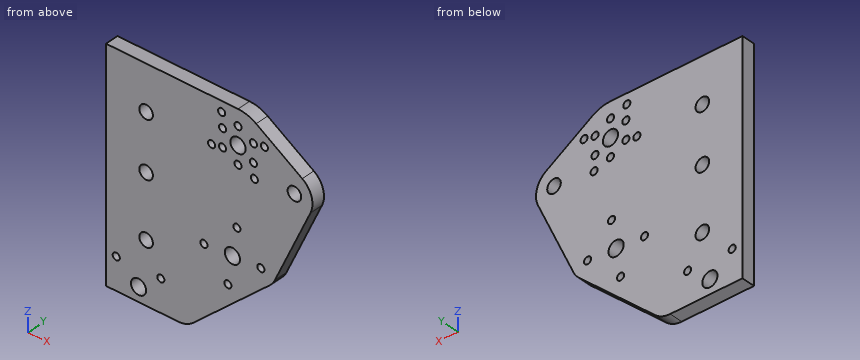
from build123d import *

# Parameters (mm, degrees)
ESBO_O1_R                = 3.4
ESBO_O1_R_2              = 1.6
ESBO_O1_R_3              = 3.05
RESSALTO_EXTRUS_O1_DEPTH = 6
ESBO_O2_R                = 3.05
CORTE_EXTRUS_O1_DEPTH    = 10


with BuildPart() as part:
    # Esboço1 → Ressalto-extrusão1 (new body)
    with BuildSketch(Plane.XZ.offset(6)):
        with BuildLine():
            ThreePointArc((148.858963728, -17.550205761), (150.213387743, -16.041631797), (151.235707119, -14.290882553))
            Line((151.235707119, -14.290882553), (167.194797105, 20.786465148))
            ThreePointArc((167.194797105, 20.786465148), (167.685761217, 27.75097204), (163.500492356, 33.339256802))
            Line((163.500492356, 33.339256802), (142.828800476, 46.629357452))
            ThreePointArc((142.828800476, 46.629357452), (138.919886426, 48.415130742), (134.666145804, 49.026919929))
            Line((134.666145804, 49.026919929), (75.43742995, 49.026919929))
            Line((75.43742995, 49.026919929), (75.43742995, -51.3))
            Line((75.43742995, -51.3), (107.856417314, -51.3))
            ThreePointArc((107.856417314, -51.3), (111.461591333, -50.627524875), (114.581887382, -48.700544058))
            Line((114.581887382, -48.700544058), (148.858963728, -17.550205761))
        make_face()
        with Locations(Location((90.03742995, -45, 0), (0, 0, 270))):
            Circle(ESBO_O1_R, mode=Mode.SUBTRACT)
        with Locations(Location((80.03742995, -37, 0), (0, 0, 270))):
            Circle(ESBO_O1_R_2, mode=Mode.SUBTRACT)
        with Locations(Location((100.03742995, -37, 0), (0, 0, 270))):
            Circle(ESBO_O1_R_2, mode=Mode.SUBTRACT)
        with Locations(Location((119.376459837, -13.805034822, 0), (0, 0, 270))):
            Circle(ESBO_O1_R_2, mode=Mode.SUBTRACT)
        with Locations(Location((130.137211947, -25.645905315, 0), (0, 0, 270))):
            Circle(ESBO_O1_R_2, mode=Mode.SUBTRACT)
        with Locations(Location((132.15737995, -13, 0), (0, 0, 270))):
            Circle(ESBO_O1_R, mode=Mode.SUBTRACT)
        with Locations(Location((144.938300063, -12.194965178, 0), (0, 0, 270))):
            Circle(ESBO_O1_R_2, mode=Mode.SUBTRACT)
        with Locations(Location((134.177547953, -0.354094685, 0), (0, 0, 270))):
            Circle(ESBO_O1_R_2, mode=Mode.SUBTRACT)
        with Locations(Location((122.816922322, 29.075437545, 0), (0, 0, 270))):
            Circle(ESBO_O1_R_2, mode=Mode.SUBTRACT)
        with Locations(Location((127.737942574, 29.932998956, 0), (0, 0, 270))):
            Circle(ESBO_O1_R_2, mode=Mode.SUBTRACT)
        with Locations(Location((134.666145804, 25.932998956, 0), (0, 0, 270))):
            Circle(ESBO_O1_R_2, mode=Mode.SUBTRACT)
        with Locations(Location((142.006279165, 23.439074893, 0), (0, 0, 270))):
            Circle(ESBO_O1_R_2, mode=Mode.SUBTRACT)
        with Locations(Location((134.666145804, 33.932998956, 0), (0, 0, 270))):
            Circle(ESBO_O1_R, mode=Mode.SUBTRACT)
        with Locations(Location((141.594349035, 29.932998956, 0), (0, 0, 270))):
            Circle(ESBO_O1_R_2, mode=Mode.SUBTRACT)
        with Locations(Location((127.737942574, 37.932998956, 0), (0, 0, 270))):
            Circle(ESBO_O1_R_2, mode=Mode.SUBTRACT)
        with Locations(Location((127.326012444, 44.426923019, 0), (0, 0, 270))):
            Circle(ESBO_O1_R_2, mode=Mode.SUBTRACT)
        with Locations(Location((134.666145804, 41.932998956, 0), (0, 0, 270))):
            Circle(ESBO_O1_R_2, mode=Mode.SUBTRACT)
        with Locations(Location((141.594349035, 37.932998956, 0), (0, 0, 270))):
            Circle(ESBO_O1_R_2, mode=Mode.SUBTRACT)
        with Locations(Location((159.995303964, 25.487660186, 0), (0, 0, 270))):
            Circle(ESBO_O1_R_3, mode=Mode.SUBTRACT)
        with Locations(Location((146.515369287, 38.790560368, 0), (0, 0, 270))):
            Circle(ESBO_O1_R_2, mode=Mode.SUBTRACT)
    extrude(amount=-RESSALTO_EXTRUS_O1_DEPTH)

    # Esboço2 → Corte-extrusão1 (cut)
    with BuildSketch(Plane.XZ.offset(6)):
        with Locations(Location((93.43742995, -24.067001044, 0), (0, 0, 270))):
            Circle(ESBO_O2_R)
        with Locations(Location((93.43742995, 3.932998956, 0), (0, 0, 270))):
            Circle(ESBO_O2_R)
        with Locations(Location((93.43742995, 28.932998956, 0), (0, 0, 270))):
            Circle(ESBO_O2_R)
    extrude(amount=-CORTE_EXTRUS_O1_DEPTH, mode=Mode.SUBTRACT)


solid = part.part
Source: CAD feature listing. Evaluate the final solid. Frame: model axes, mm. Round coordinates to 2 decimals unless told otherwise and drop trailing zeros. Write each loop counter-clockwise with the first axis right and the second up, starting at its lowest first coordinate (ties: lowest second). Pieces come first, ordered by that corner, then holes. Notation, with made-up numbers: M 55.5,6 L 107.5,6 A22 ccw 107.5,20 Z; hole C 15,-22 d10. An arc over 180 degrees is marked long. One line per item, written item: value. Start each with the question number.
Item 1: Section query A-A (z = -37). Return the cut outline in (x, y).
Item 2: Section query B-B (y = -3.9). State how many separate pieces and enclosed holes the cut face has, plus the area to 3 significant figures.
Item 3: Section query C-C (x = 154.5). Return the cut outline in (y, z).
Item 4: Pin query (flat end, axial travel): pin 1 (1.5 mm diameter, centred on x = 154.5, y = -1, fed in from -Z). Return the tip coordinate at first contact, or that it passes through.
Item 5: Ray query, L1, parallel to X at y = -1.25, z = -37; L2, parallel to X at y = -3.25, z = -26.5; L3, parallel to X at y = -2.2, z = 29. Return the intervals inside material, ascending. Write a range as from..to.
Result set:
1. outline: M 75.44,-6 L 78.44,-6 L 78.44,0 L 75.44,0 Z; M 81.64,-6 L 98.44,-6 L 98.44,0 L 81.64,0 Z; M 101.64,-6 L 127.46,-6 L 127.46,0 L 101.64,0 Z
2. separate pieces: 1
2. enclosed holes: 23
2. area: 7,020 mm²
3. outline: M -6,-7.12 L 0,-7.12 L 0,39.13 L -6,39.13 Z
4. pin 1: stops at z = -8.76
5. L1: x = 75.44..78.44, 81.64..98.44, 101.64..127.46
5. L2: x = 75.44..91.6, 95.28..128.78, 131.49..139.01
5. L3: x = 75.44..90.39, 96.49..121.22, 124.42..126.44, 129.04..140.29, 142.89..167.23
